from build123d import *

# Parameters (mm, degrees)
SKETCH1_W           = 18.5
SKETCH1_H           = 10
SKETCH1_W_2         = 5.5
SKETCH1_H_2         = 7
BOSS_EXTRUDE1_DEPTH = 1.5
SKETCH1_3_W         = 18.5
SKETCH1_3_H         = 10
SKETCH1_3_W_2       = 5.5
SKETCH1_3_H_2       = 7
BOSS_EXTRUDE2_DEPTH = 4.5
CUT_EXTRUDE1_START  = -2
SKETCH2_W           = 7
SKETCH2_H           = 0.75
CUT_EXTRUDE1_DEPTH  = 2
CUT_EXTRUDE5_START  = -16.5
SKETCH2_2_W         = 7
SKETCH2_2_H         = 0.75
CUT_EXTRUDE5_DEPTH  = 2
SKETCH4_W           = 3
SKETCH4_H           = 2.690114405
CUT_EXTRUDE3_DEPTH  = 12.437329234
CHAMFER1_SIZE       = 1
CHAMFER1_SIZE_2     = 3
FILLET2_R           = 0.5


with BuildPart() as part:
    # Sketch1 → Boss-Extrude1 (new body)
    # profile 1 of 3: a face of its own
    with BuildSketch(Plane(origin=(0, 0, 0), x_dir=(1, 0, 0), z_dir=(0, 1, 0))):
        Rectangle(SKETCH1_W, SKETCH1_H)
        with Locations((4.5, 0)):
            Rectangle(SKETCH1_W_2, SKETCH1_H_2, mode=Mode.SUBTRACT)
        with Locations((-4.5, 0)):
            Rectangle(SKETCH1_W_2, SKETCH1_H_2, mode=Mode.SUBTRACT)
    # profile 2 of 3: a face of its own
    with BuildSketch(Plane(origin=(0, 0, 0), x_dir=(1, 0, 0), z_dir=(0, 1, 0))):
        with Locations((4.5, 0)):
            Rectangle(SKETCH1_W_2, SKETCH1_H_2)
    # profile 3 of 3: a face of its own
    with BuildSketch(Plane(origin=(0, 0, 0), x_dir=(1, 0, 0), z_dir=(0, 1, 0))):
        with Locations((-4.5, 0)):
            Rectangle(SKETCH1_W_2, SKETCH1_H_2)
    extrude(amount=BOSS_EXTRUDE1_DEPTH)

    # Sketch1<3> → Boss-Extrude2 (add)
    with BuildSketch(Plane(origin=(0, 0, 0), x_dir=(1, 0, 0), z_dir=(0, 1, 0))):
        Rectangle(SKETCH1_3_W, SKETCH1_3_H)
        with Locations((-4.5, 0)):
            Rectangle(SKETCH1_3_W_2, SKETCH1_3_H_2, mode=Mode.SUBTRACT)
        with Locations((4.5, 0)):
            Rectangle(SKETCH1_3_W_2, SKETCH1_3_H_2, mode=Mode.SUBTRACT)
    extrude(amount=BOSS_EXTRUDE2_DEPTH)

    # Sketch2 → Cut-Extrude1 (cut)
    with BuildSketch(Plane.ZY.offset(9.25).offset(CUT_EXTRUDE1_START)):
        with Locations((0, 1.875)):
            Rectangle(SKETCH2_W, SKETCH2_H)
    extrude(amount=CUT_EXTRUDE1_DEPTH, mode=Mode.SUBTRACT)

    # Sketch2<2> → Cut-Extrude5 (cut)
    with BuildSketch(Plane.ZY.offset(9.25).offset(CUT_EXTRUDE5_START)):
        with Locations((0, 1.875)):
            Rectangle(SKETCH2_2_W, SKETCH2_2_H)
    extrude(amount=-CUT_EXTRUDE5_DEPTH, mode=Mode.SUBTRACT)

    # Sketch4 → Cut-Extrude3 (cut, symmetric)
    with BuildSketch(Plane(origin=(0, 0, 0), x_dir=(0, 0, 1), z_dir=(0.7071067811865488, 0.7071067811865464, 0))):
        with Locations((-2, -10.214222054)):
            Rectangle(SKETCH4_W, SKETCH4_H)
    cut_extrude3 = extrude(amount=CUT_EXTRUDE3_DEPTH, both=True, mode=Mode.SUBTRACT)

    # Sketch5 → M2 Clearance Hole1 (revolve, cut)
    with BuildSketch(Plane(origin=(-4.5, 1.5, 0), x_dir=(0, 0, 1), z_dir=(1, 0, 0))):
        Polygon((0, 0), (0, 2.321032743), (1.2, 1.6), (1.2, 0), align=None)
    m2_clearance_hole1 = revolve(axis=Axis((-4.5, 7.85, 0), (0, -1, 0)), mode=Mode.SUBTRACT)

    # Mirror4: Cut-Extrude3, M2 Clearance Hole1 across plane
    add(cut_extrude3.mirror(Plane(origin=(0, 0, 0), x_dir=(0, 0, 1), z_dir=(1, 0, 0))), mode=Mode.SUBTRACT)
    add(m2_clearance_hole1.mirror(Plane(origin=(0, 0, 0), x_dir=(0, 0, 1), z_dir=(1, 0, 0))), mode=Mode.SUBTRACT)

    # Chamfer1
    # the kernel refuses this chamfer: 3, 1 mm, written as the material it takes off along each edge
    with BuildSketch(Plane(origin=(-1.75, 4.5, -3.5), x_dir=(0.9940388851139268, 0.10902612017980688, 0), z_dir=(0, 0, 1)), Plane(origin=(1.75, 4.5, 3.5), x_dir=(-0.9940388851139268, 0.10902612017980688, 0), z_dir=(0, 0, -1))) as chamfer1_piece_1:
        Polygon((CHAMFER1_SIZE * 0.994038885114, -CHAMFER1_SIZE * 0.10902612018), (-CHAMFER1_SIZE_2 * 0.10902612018, -CHAMFER1_SIZE_2 * 0.994038885114), (0, 0), align=None)
    extrude(amount=7, mode=Mode.SUBTRACT)

    # Fillet2
    fillet2_edges = [part.edges().sort_by_distance(p)[0] for p in [
        (9.25, 4.5, -4.25),
        (1.25, 3, 3.5),
        (1.25, 3, -3.5),
        (-1.25, 3, -3.5),
        (-1.25, 3, 3.5),
        (-9.25, 4.5, -4.25),
        (9.25, 4.5, 2.25),
        (-7.25, 3.375, 3.5),
        (-7.25, 3.375, -3.5),
        (7.25, 3.375, 3.5),
        (7.25, 3.375, -3.5),
        (-9.25, 2.25, 0),
        (9.25, 2.25, 0),
        (-9.25, 4.5, 2.25),
    ]]
    fillet(fillet2_edges, radius=FILLET2_R)


solid = part.part
Design review of the part built by this model. Coordinates are the model's own, in mm. A direction names the side the tool comes from. Give positions to 0.01 mm unless a question says otherwise; leave off trailing zeros. Write each loop counter-clockwise with the first axis right and the second up, starting at its lowest first coordinate (ties: lowest second). Pieces come first, ordered by that corner, then holes. Notation, with made-up numbers: M -20,43 L -10,43 A20 cw -10,49 Z; hole C 58,-28.75 d6. An arc over 180 degrees is marked long. Return JSON: item names as keys, results as strings. Group by question number.
Item 1: Take a section at D-D (z = 2.25). Give the boundary of the cut face in (x, y), plus the area to 3 significant figures.
Item 2: Take a section at A-A (z = 0). Give the boundary of the cut face in (x, y).
Item 3: Take a section at C-C (y = 1.1). Give the boundary of the cut face in (x, z), plus the area to 3 significant figures.
Item 4: Tool access review of faces 1 (the flat face through (9, 4, -0.5)), 2 (the flat face through (-7.25, 3, 0)), 3 (the flat face through (-9, 4, -0.5)), 4 (the flat face through (6, 1.5, 0)): name each direction out of +Z, -Z, +X, -X, +Y, -Y from which nothing blocks a thin tool from reaching the whole face with its end or side.
Item 5: Clearance check with a flat-ended pin moving along its axis: pin 1 Ø3 at (x, z) = (4.5, 0) entering from +Y. State where the tip first meets the part, or that it passes through.
Item 6: Wall thickness on line 1 along X through (y, z) = (0.55, 0); line 2 along Z through (x, y) = (-4.5, 0.5); line 3 along X through (y, z) = (3.65, 0.5): over which ranges is each line inside the solid? List them lowest first.
Item 7: Take a section at B-B (x = 4.5). Give the boundary of the cut face in (y, z), plus the area to 3 significant figures.
Item 8: The part is to be moulded in two halves that separate along Y. For faces 5 (the cylindrical face through (5.51, 0.76, 0.65)), 6 (the flat face through (1.243, 3.021, 0.042)), 7 (the flat face through (-8, 2.25, 0)), say which applies: pulls with the +Y half, pulls with the -Y half, needs draft (parallel to the pull), parting line crosses it, or undercut.
Return value:
{
 "1": {"outline": "M -9.25,0 L 9.25,0 L 9.25,1.5 L 1.75,1.5 L 0.75,4.5 L -0.75,4.5 L -1.75,1.5 L -9.25,1.5 Z; M -9.25,2.75 A0.5 ccw -8.75,2.25 L -7.25,2.25 L -7.25,4.5 L -8.75,4.5 A0.5 ccw -9.25,4 Z; M 7.25,2.25 L 8.75,2.25 A0.5 ccw 9.25,2.75 L 9.25,4 A0.5 ccw 8.75,4.5 L 7.25,4.5 Z", "area": "44.0 mm2"},
 "2": {"outline": "M -9.25,0 L -5.7,0 L -5.7,1.5 L -9.25,1.5 Z; M -9.25,2.75 A0.5 ccw -8.75,2.25 L -7.25,2.25 L -7.25,4.5 L -8.75,4.5 A0.5 ccw -9.25,4 Z; M -3.3,0 L 3.3,0 L 3.3,1.5 L 1.75,1.5 L 0.75,4.5 L -0.75,4.5 L -1.75,1.5 L -3.3,1.5 Z; M 5.7,0 L 9.25,0 L 9.25,1.5 L 5.7,1.5 Z; M 7.25,2.25 L 8.75,2.25 A0.5 ccw 9.25,2.75 L 9.25,4 A0.5 ccw 8.75,4.5 L 7.25,4.5 Z"},
 "3": {"outline": "M -9.25,-5 L 9.25,-5 L 9.25,5 L -9.25,5 Z; hole C -4.5,0 d2.4; hole C 4.5,0 d2.4", "area": "176 mm2"},
 "4": {"face 1": "+X, +Y", "face 2": "+Y", "face 3": "-X, +Y", "face 4": "+X"},
 "5": {"pin 1": "stops at y = 1.5"},
 "6": {"line 1": "x = -9.25 to -5.7, -3.3 to 3.3, 5.7 to 9.25", "line 2": "z = -5 to -1.2, 1.2 to 5", "line 3": "x = -9.25 to -7.25, -1.03 to 1.03, 7.25 to 9.25"},
 "7": {"outline": "M 0,-5 L 4.5,-5 L 4.5,-3.5 L 1.5,-3.5 L 1.5,-1.2 L 0,-1.2 Z; M 0,1.2 L 1.5,1.2 L 1.5,3.5 L 4.5,3.5 L 4.5,5 L 0,5 Z", "area": "20.4 mm2"},
 "8": {"face 5": "needs draft", "face 6": "pulls with the +Y half", "face 7": "undercut"}
}
